Source: CAD feature listing. Evaluate the final solid. Frame: model axes, mm. A direction names the side the tool comes from. Round coordinates to 2 decimals unless told otherwise and drop trailing zeros. Loops run counter-clockwise (first coordinate to the right, second up) from the corner with the lowest first, then second, coordinate; pieces in that order, holes last. Notation, with made-up numbers: (18, -7.75) -> (64, -7.75) arc R33 cw to (64, 28.25) -> close; hole circle Ø8 at (85, -40). An arc over 180 degrees is marked (long way). Put each result on its own line as item: value. Start each with the question number.
1. Set-up query: faces 1 (the flat face through (-136.09, -0.9, -294.95)), 2 (the flat face through (-135.86, -0.9, 295.18)), 3 (the flat face through (-295.18, -0.9, -135.86)). Return all of +Z, -Z, +X, -X, +Y, -Y with unobstructed straight access to the full face (end or side cutting, diameter ignored); none if empty.
2. Contact query for flat-ended pins moving along their axis: pin 1 (0.9 mm diameter, centred on x = -107, y = -1, fed in from +Z); pin 2 (0.9 mm diameter, centred on x = 307.5, y = -1, fed in from -Z); pin 3 (0.5 mm diameter, centred on x = 309.5, y = -0.5, fed in from +Z). Output: stop coordinate, or through.
3. Cut plane A-A (x = -41.5). Return the cut outline in (y, z).
4. Cut plane C-C (y = -1.45). State how many separate pieces and enclosed holes the cut face has, then the cut area to 3 significant figures.
5. Cut plane B-B (z = -54). Return the cut outline in (x, y).
6. Material intervals for L1, parallel to X at y = -0.7, z = 160; L2, parallel to X at y = -1.05, z = -179.5; L3, parallel to Z at x = 294.5, y = -0.25, sorted ascending.
7. Draft query along Z for faces 4 (the flat face through (-4, 0, -67)), 5 (the flat face through (295.18, -0.9, 135.86)), 6 (the flat face through (136.09, -0.9, 294.95)). Return one class per face: pulls with the +Z half, pulls with the -Z half, needs draft (parallel to the pull), parting line crosses it, or undercut.
```python
from build123d import *

# Parameters (mm, degrees)
F0_R     = 3.175
F0_R_2   = 6.35
F1_DEPTH = 1.8288
F2_R     = 5.08


with BuildPart() as f1:
    # F0 (on Front) → F1 (new body)
    with BuildSketch(Plane.XZ):
        Polygon((-100.838, 304.8), (-126.238, 304.8), (-144.215766, 286.822234), (-155.448233, 298.054701), (-182.389002, 271.113932), (-171.156535, 259.881465), (-259.881465, 171.156535), (-271.113932, 182.389002), (-298.054701, 155.448233), (-286.822234, 144.215766), (-304.8, 126.238), (-304.8, 100.838), (-320.675, 100.838), (-320.675, 62.738), (-304.8, 62.738), (-304.8, -62.738), (-320.675, -62.738), (-320.675, -100.838), (-304.8, -100.838), (-304.8, -126.238), (-286.822234, -144.215766), (-298.054701, -155.448233), (-271.113932, -182.389002), (-259.881465, -171.156535), (-171.156535, -259.881465), (-182.389002, -271.113932), (-155.448233, -298.054701), (-144.215766, -286.822234), (-126.238, -304.8), (-100.838, -304.8), (-100.838, -320.675), (-62.738, -320.675), (-62.738, -304.8), (62.738, -304.8), (62.738, -320.675), (100.838, -320.675), (100.838, -304.8), (126.238, -304.8), (144.215766, -286.822234), (155.448233, -298.054701), (182.389002, -271.113932), (171.156535, -259.881465), (259.881465, -171.156535), (271.113932, -182.389002), (298.054701, -155.448233), (286.822234, -144.215766), (304.8, -126.238), (304.8, -100.838), (320.675, -100.838), (320.675, -62.738), (304.8, -62.738), (304.8, 62.738), (320.675, 62.738), (320.675, 100.838), (304.8, 100.838), (304.8, 126.238), (286.822234, 144.215766), (298.054701, 155.448233), (271.113932, 182.389002), (259.881465, 171.156535), (171.156535, 259.881465), (182.389002, 271.113932), (155.448233, 298.054701), (144.215766, 286.822234), (126.238, 304.8), (100.838, 304.8), (100.838, 320.675), (62.738, 320.675), (62.738, 304.8), (-62.738, 304.8), (-62.738, 320.675), (-100.838, 320.675), align=None)
        with Locations((-162.614478, -278.280177)):
            Circle(F0_R, mode=Mode.SUBTRACT)
        with Locations((-278.280177, -162.614478)):
            Circle(F0_R, mode=Mode.SUBTRACT)
        with Locations((-81.788, -311.7596)):
            Circle(F0_R, mode=Mode.SUBTRACT)
        with Locations((-311.7596, -81.788)):
            Circle(F0_R, mode=Mode.SUBTRACT)
        with Locations((81.788, -311.7596)):
            Circle(F0_R, mode=Mode.SUBTRACT)
        with Locations((162.614478, -278.280177)):
            Circle(F0_R, mode=Mode.SUBTRACT)
        with Locations((278.280177, -162.614478)):
            Circle(F0_R, mode=Mode.SUBTRACT)
        with Locations((311.7596, -81.788)):
            Circle(F0_R, mode=Mode.SUBTRACT)
        with Locations((-311.7596, 81.788)):
            Circle(F0_R, mode=Mode.SUBTRACT)
        with Locations((-278.280177, 162.614478)):
            Circle(F0_R, mode=Mode.SUBTRACT)
        with Locations((-162.614478, 278.280177)):
            Circle(F0_R, mode=Mode.SUBTRACT)
        with Locations((-81.788, 311.7596)):
            Circle(F0_R, mode=Mode.SUBTRACT)
        Circle(F0_R_2, mode=Mode.SUBTRACT)
        with Locations((311.7596, 81.788)):
            Circle(F0_R, mode=Mode.SUBTRACT)
        with Locations((81.788, 311.7596)):
            Circle(F0_R, mode=Mode.SUBTRACT)
        with Locations((278.280177, 162.614478)):
            Circle(F0_R, mode=Mode.SUBTRACT)
        with Locations((162.614478, 278.280177)):
            Circle(F0_R, mode=Mode.SUBTRACT)
    extrude(amount=F1_DEPTH)

    # F2
    f2_edges = [f1.edges().sort_by_distance(p)[0] for p in [
        (-271.113932, -0.9144, 182.389002),
        (-298.054701, -0.9144, 155.448233),
        (-182.389002, -0.9144, 271.113932),
        (-155.448233, -0.9144, 298.054701),
        (-100.838, -0.9144, 320.675),
        (-62.738, -0.9144, 320.675),
        (62.738, -0.9144, 320.675),
        (100.838, -0.9144, 320.675),
        (155.448233, -0.9144, 298.054701),
        (182.389002, -0.9144, 271.113932),
        (271.113932, -0.9144, 182.389002),
        (298.054701, -0.9144, 155.448233),
        (320.675, -0.9144, 100.838),
        (320.675, -0.9144, 62.738),
        (320.675, -0.9144, -62.738),
        (320.675, -0.9144, -100.838),
        (298.054701, -0.9144, -155.448233),
        (271.113932, -0.9144, -182.389002),
        (182.389002, -0.9144, -271.113932),
        (155.448233, -0.9144, -298.054701),
        (100.838, -0.9144, -320.675),
        (62.738, -0.9144, -320.675),
        (-62.738, -0.9144, -320.675),
        (-100.838, -0.9144, -320.675),
        (-155.448233, -0.9144, -298.054701),
        (-182.389002, -0.9144, -271.113932),
        (-271.113932, -0.9144, -182.389002),
        (-298.054701, -0.9144, -155.448233),
        (-320.675, -0.9144, -100.838),
        (-320.675, -0.9144, -62.738),
        (-320.675, -0.9144, 62.738),
        (-320.675, -0.9144, 100.838),
        (126.238, -0.9144, 304.8),
        (304.8, -0.9144, 126.238),
        (304.8, -0.9144, -126.238),
        (126.238, -0.9144, -304.8),
        (-126.238, -0.9144, -304.8),
        (-304.8, -0.9144, -126.238),
        (-304.8, -0.9144, 126.238),
        (-126.238, -0.9144, 304.8),
    ]]
    fillet(f2_edges, radius=F2_R)


solid = f1.part
```
Solution:
1. face 1: -Z, +Y, -Y
1. face 2: +Z, +Y, -Y
1. face 3: -X, +Y, -Y
2. pin 1: stops at z = 304.8
2. pin 2: stops at z = -100.84
2. pin 3: stops at z = 100.84
3. outline: (-1.83, -304.8) -> (0, -304.8) -> (0, 304.8) -> (-1.83, 304.8) -> close
4. separate pieces: 1
4. enclosed holes: 17
4. area: 317,000 mm^2
5. outline: (-304.8, -1.83) -> (304.8, -1.83) -> (304.8, 0) -> (-304.8, 0) -> close
6. L1: x = -293.5 to -280.08, -276.48 to 276.48, 280.08 to 293.5
6. L2: x = -273.83 to -268.4, -251.54 to 251.54, 268.4 to 273.83
6. L3: z = -159 to -151.89, -136.54 to 136.54, 151.89 to 159
7. face 4: needs draft
7. face 5: undercut
7. face 6: pulls with the +Z half
